Check sheet for the modelled part. Datum: model origin and axes. Units: mm. Face numbers are marked on the shaded views. Coordinates: 2 decimals unless noted, no trailing zeros. Loops run counter-clockwise (first coordinate to the right, second up) from the corner with the lowest first, then second, coordinate; pieces in that order, holes last. Notation, with made-up numbers: (33.25, 85) -> (47.25, 85) arc R8 cw to (47.25, 100) -> close; hole circle Ø4 at (48, -29). An arc over 180 degrees is marked (long way). Use CSV: the item, a comma, the result in double quotes. Start each with the question number.
1. Sectioned sample at C-C, the plane x = -40. Record the cut outline in (y, z).
2. Sectioned sample at A-A, the plane x = 67. Record the cut outline in (y, z), and give its area (3 significant figures).
3. Gauge pin test, flat ends, axial feed: pin 1 (2.5 mm diameter, centred on x = -10.5, z = -18, fed in from +Y); pin 2 (4 mm diameter, centred on y = 2, z = 9, fed in from +X); pin 3 (9.5 mm diameter, centred on x = 43, z = 1.5, fed in from +Y); pin 4 (4 mm diameter, centred on x = -67, z = 0, fed in from -Y). Record the tip position at first contact, or that the pin passes through.
4. Release check for a two-part mould opening along Z. For the marked faces 1 and 2 record: pulls with the +Z half, pulls with the -Z half, needs draft (parallel to the pull), parting line crosses it, or undercut.
5. Thickness scan on L1, parallel to Z at x = -3.5, y = 11; L2, parallel to Z at x = 40, y = 7.5; L3, parallel to Z at x = 67, y = 10.05. Record the ranges inside material, lowest first.
6. Sectioned sample at B-B, the plane z = 0. Count the separate pieces of the cut face and the enclosed holes in it, and give its area (3 significant figures).
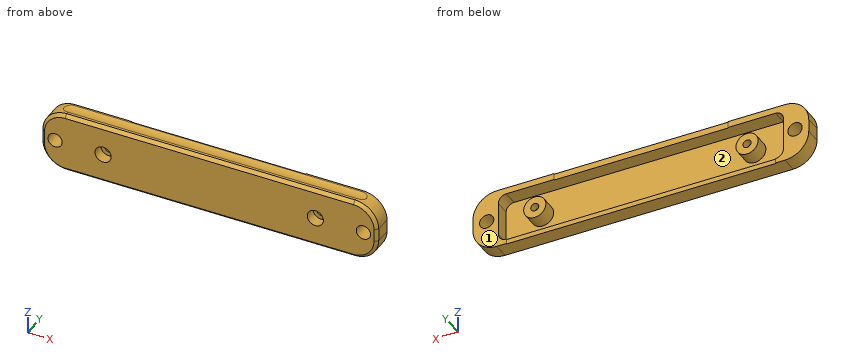
Autodesk Inventor part; units mm, degrees
ref_plane "YZ Plane" through (0, 0, 0) normal (1, 0, 0) x (0, 1, 0)
ref_plane "XZ Plane" through (0, 0, 0) normal (0, 1, 0) x (-1, 0, 0)
ref_plane "XY Plane" through (0, 0, 0) normal (0, 0, 1) x (1, 0, 0)
sketch "Body Outline" plane through (0, 0, 0) normal (0, 1, 0) x (-1, 0, 0)
  line L0 (106, -19) -> (-106, -19)
  line L1 (-106, -19) -> (-106, 19)
  line L2 (-106, 19) -> (106, 19)
  line L3 (106, 19) -> (106, -19)
  point P0 (0, 0)
  dimension "d0" = 38
  dimension "d1" = 19
  dimension "d2" = 212
  dimension "d3" = 106
extrude "Body" add sketch "Body Outline" along normal blind 12
sketch "Body Cutout Outline" plane through (0, 12, 0) normal (0, 1, 0) x (1, 0, 0)
  line L0 (-90, -15) -> (90, -15)
  line L1 (90, -15) -> (90, 16)
  line L2 (90, 16) -> (-90, 16)
  line L3 (-90, 16) -> (-90, -15)
  circle A0 centre (-67, 0) radius 7
  circle A1 centre (67, 0) radius 7
  line L4 (-106, -19) -> (106, -19)
  point P0 (0, 0)
  dimension "d6" = 31
  dimension "d8" = 180
  dimension "d9" = 90
  dimension "d12" = 14
  dimension "d13" = 14
  dimension "d14" = 0
  dimension "d15" = 67
  dimension "d16" = 67
  dimension "d17" = 0
  dimension "d68" = 4
extrude "Body Cutout" cut sketch "Body Cutout Outline" against normal blind 9.5
sketch "Skin Passages Outline" plane through (0, 12, 0) normal (0, 1, 0) x (1, 0, 0)
  line L0 (-85, 16) -> (85, 16)
  line L1 (85, 16) -> (85, 19)
  line L2 (85, 19) -> (-85, 19)
  line L3 (-85, 19) -> (-85, 16)
  line L4 (106, 19) -> (-106, 19)
  line L5 (-55, -19) -> (55, -19)
  line L6 (55, -19) -> (55, -15)
  line L7 (55, -15) -> (-55, -15)
  line L8 (-55, -15) -> (-55, -19)
  line L9 (-106, -19) -> (106, -19)
  point P0 (0, 0)
  dimension "d20" = 0
  dimension "d21" = 3
  dimension "d22" = 170
  dimension "d23" = 85
  dimension "d24" = 0
  dimension "d25" = 4
  dimension "d26" = 110
  dimension "d27" = 55
extrude "Skin Passages" cut sketch "Skin Passages Outline" against normal blind 0.5
sketch "Fastening Hole Positions" plane through (0, 0, 0) normal (0, -1, 0) x (1, 0, 0)
  point P0 (0, 0)
  point P1 (67, 0)
  point P2 (-67, 0)
  dimension "d30" = 67
  dimension "d31" = 67
  dimension "d32" = 0
  dimension "d33" = 0
hole "Fastening Holes" at (67, 0, 0) at (-67, 0, 0) direction (0, 1, 0) diameter 5.1 end through all counterbore diameter 10.2 counterbore depth 7
sketch "Thumbscrew Hole Positions" plane through (0, 0, 0) normal (0, -1, 0) x (1, 0, 0)
  circle A0 centre (-97.35, 0) radius 4.5
  circle A1 centre (97.35, 0) radius 4.5
  line L0 (106, -19) -> (106, 19)
  line L1 (-106, 19) -> (-106, -19)
  point P0 (0, 0)
  dimension "d44" = 9
  dimension "d45" = 9
  dimension "d47" = 0
  dimension "d49" = 0
  dimension "d66" = 8.65
  dimension "d67" = 8.65
extrude "Thumbscrew Holes" cut sketch "Thumbscrew Hole Positions" along normal through all both and the other way through all
sketch "Side Cutout Outline" plane through (-106, 0, -19) normal (-1, 0, 0) x (0, 0, 1)
  circle A0 centre (47.3, 7.25) radius 10
  line L0 (38, 0) -> (38, 12)
  line L1 (0, 12) -> (38, 12)
  point P0 (19, 0)
  dimension "d69" = 20
  dimension "d70" = 9.3
  dimension "d71" = 4.75
extrude "Side Cutout" cut sketch "Side Cutout Outline" along normal through all both and the other way through all
fillet "Body Fillet" radius 5 4 edges at (-90, 7.25, -16) (90, 7.25, -16) (90, 7.25, 15) (-90, 7.25, 15)
fillet "Body Fillet" radius 15 4 edges at (-106, 1.7872, 19) (-106, 6, -19) (106, 6, -19) (106, 1.7872, 19)
chamfer "Body Chamfer" distance 2 angle 45 4 edges at (0, 0, 19) (106, 0, 0) (0, 0, -19) (-106, 0, 0)
properties part number "LR Top Cover Studs End" material "Acetal Resin, Black"
Completed:
1,outline,"(0, -17) -> (2, -19) -> (11.5, -19) -> (11.5, -16) -> (2.5, -16) -> (2.5, 15) -> (11.5, 15) -> (11.5, 19) -> (10.93, 19) arc R10 cw to (3.57, 19) -> (2, 19) -> (0, 17) -> close"
2,outline,"(0, -17) -> (2, -19) -> (11.5, -19) -> (11.5, -16) -> (2.5, -16) -> (2.5, -7) -> (12, -7) -> (12, -2.55) -> (7, -2.55) -> (7, -5.1) -> (0, -5.1) -> close; (0, 5.1) -> (7, 5.1) -> (7, 2.55) -> (12, 2.55) -> (12, 7) -> (2.5, 7) -> (2.5, 15) -> (12, 15) -> (12, 19) -> (10.93, 19) arc R10 cw to (3.57, 19) -> (2, 19) -> (0, 17) -> close"
2,area,"189 mm²"
3,pin 1,"y = 11.5"
3,pin 2,"x = 105.7"
3,pin 3,"y = 2.5"
3,pin 4,"through"
4,face 1,"needs draft"
4,face 2,"undercut"
5,L1,"-19 to -16, 15 to 19"
5,L2,"-19 to -16, 15 to 18.3"
5,L3,"-19 to -16, -7 to -2.55, 2.55 to 7, 15 to 18.7"
6,separate pieces,"5"
6,enclosed holes,"0"
6,area,"686 mm²"
